The model under review builds one solid part; all positions refer to its coordinate system, in mm. Coordinates: 2 decimals unless noted, no trailing zeros. Order: outer loops, then holes, each group sorted by start corner. A loop starts at its lowest first (then second) coordinate and runs counter-clockwise, first axis right, second up. Notation, with made-up numbers: M 41.25,61 L 78.25,61 A11 cw 78.25,70 Z; hole C 85,-28 d1. An arc over 180 degrees is marked long. One line per item, written item: value.
```python
from build123d import *

# Parameters (mm, degrees)
SKETCH2_R           = 7.75
SKETCH2_R_2         = 2.9
SKETCH2_R_3         = 2
BOSS_EXTRUDE1_DEPTH = 5
FILLET1_R           = 2
FILLET2_R           = 2


with BuildPart() as part:
    # Sketch2 → Boss-Extrude1 (new body)
    with BuildSketch(Plane(origin=(0, 0, 0), x_dir=(1, 0, 0), z_dir=(0, 1, 0))):
        with BuildLine():
            Line((-36, 12), (-36, 36))
            Line((-36, 36), (36, 36))
            Line((36, 36), (36, 12))
            Line((36, 12), (23, 12))
            ThreePointArc((23, 12), (11, 0), (23, -12))
            Line((23, -12), (36, -12))
            Line((36, -12), (36, -36))
            Line((36, -36), (-36, -36))
            Line((-36, -36), (-36, -12))
            Line((-36, -12), (-23, -12))
            ThreePointArc((-23, -12), (-11, 0), (-23, 12))
            Line((-23, 12), (-36, 12))
        make_face()
        with Locations(Location((0, 0, 0), (0, 0, 270))):
            Circle(SKETCH2_R, mode=Mode.SUBTRACT)
        with Locations(Location((-27, 27, 0), (0, 0, 270))):
            Circle(SKETCH2_R_2, mode=Mode.SUBTRACT)
        with Locations(Location((27, 27, 0), (0, 0, 270))):
            Circle(SKETCH2_R_2, mode=Mode.SUBTRACT)
        with Locations(Location((27, -27, 0), (0, 0, 270))):
            Circle(SKETCH2_R_2, mode=Mode.SUBTRACT)
        with Locations(Location((-27, -27, 0), (0, 0, 270))):
            Circle(SKETCH2_R_2, mode=Mode.SUBTRACT)
        with Locations(Location((0, -27, 0), (0, 0, 270))):
            Circle(SKETCH2_R_3, mode=Mode.SUBTRACT)
        with Locations(Location((0, 27, 0), (0, 0, 270))):
            Circle(SKETCH2_R_3, mode=Mode.SUBTRACT)
    extrude(amount=BOSS_EXTRUDE1_DEPTH)

    # Fillet1
    fillet1_edges = [part.edges().sort_by_distance(p)[0] for p in [
        (36, 2.5, 36),
        (-36, 2.5, 36),
        (-36, 2.5, -36),
        (36, 2.5, -36),
    ]]
    fillet(fillet1_edges, radius=FILLET1_R)

    # Fillet2
    fillet2_edges = [part.edges().sort_by_distance(p)[0] for p in [
        (36, 2.5, -12),
        (36, 2.5, 12),
        (-36, 2.5, 12),
        (-36, 2.5, -12),
    ]]
    fillet(fillet2_edges, radius=FILLET2_R)


solid = part.part
```
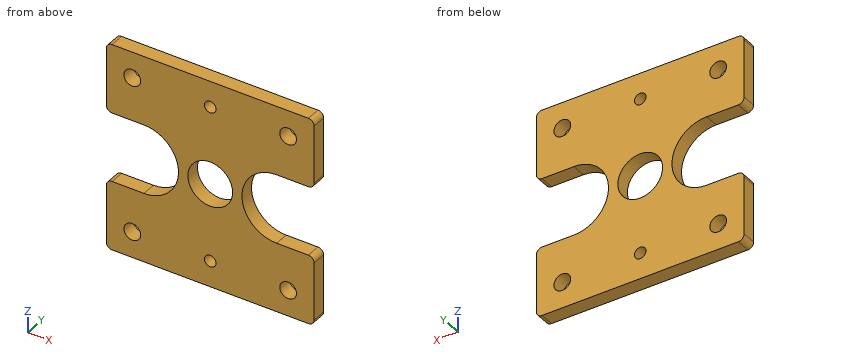
(1) We need section D-D, the plane z = -27. State the section outline as (x, y) points.
Geometry results:
outline: M -36,0 L -29.9,0 L -29.9,5 L -36,5 Z; M -24.1,0 L -2,0 L -2,5 L -24.1,5 Z; M 2,0 L 24.1,0 L 24.1,5 L 2,5 Z; M 29.9,0 L 36,0 L 36,5 L 29.9,5 Z
(2) We need section B-B, the plane z = 0. State the section outline as (x, y) points.
Geometry results:
outline: M -11,0 L -7.75,0 L -7.75,5 L -11,5 Z; M 7.75,0 L 11,0 L 11,5 L 7.75,5 Z
(3) For L1, parallel to X at y = 1.7, z = -27; L2, parallel to Z at x = 31, y = 2.4; L3, parallel to X at y = 1.35, z = 0, list the stretches that pass through material, from the lowest coordinate up.
Geometry results:
L1: x = -36 to -29.9, -24.1 to -2, 2 to 24.1, 29.9 to 36
L2: z = -36 to -12, 12 to 36
L3: x = -11 to -7.75, 7.75 to 11
(4) Insertion check: pin 1 Ø4.5 at (x, z) = (-27, -27) entering from -Y. The pin has a flat end and moves straight along its axis. Give the tip position at first contact, or say it passes through.
Geometry results:
pin 1: passes through
(5) We need section C-C, the plane y = 2.2. State the section outline as (x, z) points, plus the area to 3 significant figures.
Geometry results:
outline: M -36,-34 A2 ccw -34,-36 L 34,-36 A2 ccw 36,-34 L 36,-14 A2 ccw 34,-12 L 23,-12 A12 cw 23,12 L 34,12 A2 ccw 36,14 L 36,34 A2 ccw 34,36 L -34,36 A2 ccw -36,34 L -36,14 A2 ccw -34,12 L -23,12 A12 cw -23,-12 L -34,-12 A2 ccw -36,-14 Z; hole C -27,-27 d5.8; hole C -27,27 d5.8; hole C 0,0 d15.5; hole C 0,-27 d4; hole C 0,27 d4; hole C 27,-27 d5.8; hole C 27,27 d5.8
area: 3,780 mm2
(6) We need section A-A, the plane x = 0. State the section outline as (y, z) points, plus the area to 4 significant figures.
Geometry results:
outline: M 0,-36 L 5,-36 L 5,-29 L 0,-29 Z; M 0,-25 L 5,-25 L 5,-7.75 L 0,-7.75 Z; M 0,7.75 L 5,7.75 L 5,25 L 0,25 Z; M 0,29 L 5,29 L 5,36 L 0,36 Z
area: 242.5 mm2
